```python
from build123d import *

# Parameters (mm, degrees)
SKETCH_1_W      = 18
SKETCH_1_H      = 30
SKETCH_1_R      = 2.65
EXTRUDE_1_DEPTH = 3
SKETCH_2_W      = 18
SKETCH_2_H      = 20
EXTRUDE_2_DEPTH = 3
FILLET_1_R      = 2
EXTRUDE_3_DEPTH = 3
EXTRUDE_4_DEPTH = 3
FILLET_2_R      = 2


with BuildPart() as part:
    # 草图1 → 凸台-拉伸1 (new body)
    with BuildSketch(Plane.XY):
        with Locations((9, -15)):
            Rectangle(SKETCH_1_W, SKETCH_1_H)
        with Locations((9, -6)):
            Circle(SKETCH_1_R, mode=Mode.SUBTRACT)
        with Locations((9, -21)):
            Circle(SKETCH_1_R, mode=Mode.SUBTRACT)
    extrude(amount=EXTRUDE_1_DEPTH)

    # 草图2 → 凸台-拉伸2 (add)
    with BuildSketch(Plane(origin=(0, -30, 0), x_dir=(-1, 0, 0), z_dir=(0, -1, 0))):
        with Locations((-9, 10)):
            Rectangle(SKETCH_2_W, SKETCH_2_H)
        with BuildLine():
            Line((-10.6, 6.025104147), (-10.6, 16.025104147))
            ThreePointArc((-10.6, 16.025104147), (-9, 17.625104147), (-7.4, 16.025104147))
            Line((-7.4, 16.025104147), (-7.4, 6.025104147))
            ThreePointArc((-7.4, 6.025104147), (-9, 4.425104147), (-10.6, 6.025104147))
        make_face(mode=Mode.SUBTRACT)
    extrude(amount=-EXTRUDE_2_DEPTH)

    # 圆角1
    fillet_1_edges = [part.edges().sort_by_distance(p)[0] for p in [
        (0, -28.5, -20),
        (18, -28.5, -20),
        (0, 0, 1.5),
        (18, 0, 1.5),
    ]]
    fillet(fillet_1_edges, radius=FILLET_1_R)

    # 草图3 → 凸台-拉伸3 (add)
    with BuildSketch(Plane.ZY):
        Polygon((0, -9.628512941), (-19.146125, -27), (0, -27), align=None)
    extrude(amount=-EXTRUDE_3_DEPTH)

    # 草图4 → 凸台-拉伸4 (add)
    with BuildSketch(Plane(origin=(18, 0, 0), x_dir=(0, 0, -1), z_dir=(1, 0, 0))):
        Polygon((0, -9.628512941), (19.146125, -27), (0, -27), align=None)
    extrude(amount=-EXTRUDE_4_DEPTH)

    # 圆角2
    fillet_2_edges = [part.edges().sort_by_distance(p)[0] for p in [
        (1.5, -9.628512941, 0),
        (1.680488334, -27, -19.146125),
        (16.319511666, -27, -19.146125),
        (16.5, -9.628512941, 0),
        (9, -30, 3),
    ]]
    fillet(fillet_2_edges, radius=FILLET_2_R)


solid = part.part
```
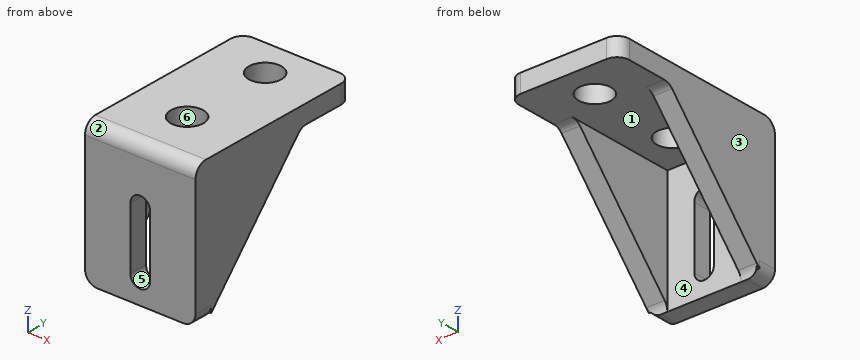
Design review of the part built by this model. Coordinates are the model's own, in mm. Face numbers are marked on the shaded views. A direction names the side the tool comes from. Coordinates: 2 decimals unless noted, no trailing zeros. Loops run counter-clockwise (first coordinate to the right, second up) from the corner with the lowest first, then second, coordinate; pieces in that order, holes last.
Q1. For pin 1 (3 mm diameter, centred on x = 6.5, z = -9, fed in from +Y), flat-tipped, find the tip position at first contact; note if it passes through.
Reported:
pin 1: stops at y = -27
Q2. We need section A-A on y = -6. State the section outline as (x, z) points, and give its area (3 significant figures).
Reported:
outline: (0, 0) - (6.35, 0) - (6.35, 3) - (0, 3) - close; (11.65, 0) - (18, 0) - (18, 3) - (11.65, 3) - close
area: 38.1 mm2
Q3. To check wall thickness, follow line 1 (Y direction, x = 9, z = 0.85); line 2 (Y direction, x = 9, z = 1.75); line 3 (X direction, y = -14, z = -3). State the ranges of each line that lie inside material, in increasing order.
Reported:
line 1: y = -30 to -23.65, -18.35 to -8.65, -3.35 to 0
line 2: y = -29.85 to -23.65, -18.35 to -8.65, -3.35 to 0
line 3: x = 0 to 3, 15 to 18
Q4. We need section C-C on z = -17. State the section outline as (x, y) points.
Reported:
outline: (0, -30) - (7.73, -30) - (7.73, -27) - (3, -27) - (3, -25.05) - (0, -25.05) - close; (10.27, -30) - (18, -30) - (18, -25.05) - (15, -25.05) - (15, -27) - (10.27, -27) - close
Q5. The part is to be moulded in two halves that separate along X. For the marked faces 1, 2 and 3, say which applies: +X half, -X half, draft (parallel to the pull), parting line (faces both ways), or undercut.
Reported:
face 1: undercut
face 2: draft
face 3: -X half
Q6. Tool access review of the marked faces 4, 5 and 6: name each direction out of +Z, -Z, +X, -X, +Y, -Y from which nothing blocks a thin tool from reaching the whole face with its end or side.
Reported:
face 4: -Z, +Y
face 5: +Y, -Y
face 6: +Z, -Z
Q7. We need section B-B on x = 9. State the section outline as (y, z) points.
Reported:
outline: (-30, -20) - (-27, -20) - (-27, -17.63) - (-30, -17.63) - close; (-30, -4.43) - (-27, -4.43) - (-27, 0) - (-23.65, 0) - (-23.65, 3) - (-28, 3) arc R2 ccw to (-30, 1) - close; (-18.35, 0) - (-8.65, 0) - (-8.65, 3) - (-18.35, 3) - close; (-3.35, 0) - (0, 0) - (0, 3) - (-3.35, 3) - close
Q8. We need section D-D on z = -4. State the section outline as (x, y) points, and give its area (3 significant figures).
Reported:
outline: (0, -30) - (18, -30) - (18, -13.26) - (15, -13.26) - (15, -27) - (3, -27) - (3, -13.26) - (0, -13.26) - close
area: 136 mm2
